Autodesk Inventor part; units mm, degrees
ref_plane "YZ Plane" through (0, 0, 0) normal (1, 0, 0) x (0, 1, 0)
ref_plane "XZ Plane" through (0, 0, 0) normal (0, 1, 0) x (-1, 0, 0)
ref_plane "XY Plane" through (0, 0, 0) normal (0, 0, 1) x (1, 0, 0)
sketch "Sketch1" plane through (0, 0, 0) normal (0, 0, 1) x (1, 0, 0)
  circle A0 centre (0, 0) radius 37.7825
  dimension "d0" = 75.565
extrude "Extrusion1" add sketch "Sketch1" against normal blind 6.35
sketch "Sketch2" plane through (0, 0, 0) normal (0, 0, 1) x (1, 0, 0)
  line L0 (-31.115, -10.4775) -> (31.115, -10.4775)
  line L1 (31.115, -10.4775) -> (31.115, -17.6657)
  line L2 (31.115, -17.6657) -> (-31.115, -17.6657)
  line L3 (-31.115, -17.6657) -> (-31.115, -10.4775)
  line L4 (-31.115, 15.5575) -> (31.115, 15.5575)
  line L5 (31.115, 15.5575) -> (31.115, 10.4775)
  line L6 (31.115, 10.4775) -> (-31.115, 10.4775)
  line L7 (-31.115, 10.4775) -> (-31.115, 15.5575)
  point P0 (0, 0)
  point P1 (31.115, -14.0716)
  point P2 (31.115, 13.0175)
  dimension "d3" = 7.1882
  dimension "d4" = 62.23
  dimension "d5" = 31.115
  dimension "d6" = 10.4775
  dimension "d10" = 62.23
  dimension "d11" = 31.115
  dimension "d12" = 10.4775
  dimension "d13" = 5.08
extrude "Extrusion2" add sketch "Sketch2" along normal blind 119.38
fillet "Fillet1" radius 3.175 5 edges at (-31.115, -14.0716, 119.38) (31.115, -14.0716, 119.38) (31.115, -17.6657, 59.69) (-31.115, -17.6657, 59.69) (0, -17.6657, 119.38)
fillet "Fillet2" radius 3.175 5 edges at (-31.115, 13.0175, 119.38) (31.115, 13.0175, 119.38) (-31.115, 15.5575, 59.69) (0, 15.5575, 119.38) (31.115, 15.5575, 59.69)
sketch "Sketch3" plane through (-31.115, -10.4775, 0) normal (0, 1, 0) x (1, 0, 0)
  line L0 (0, -116.205) -> (0, 0)
  line L1 (59.055, -119.38) -> (3.175, -119.38)
  line L2 (62.23, 0) -> (62.23, -116.205)
  line L3 (59.055, 0) -> (3.175, 0)
  point P0 (31.115, 0)
  point P1 (7.5438, -111.8362)
  point P2 (7.5438, -7.5438)
  point P3 (54.6862, -7.5438)
  point P4 (54.6862, -111.8362)
  dimension "d15" = 7.5438
  dimension "d16" = 7.5438
  dimension "d17" = 7.5438
  dimension "d18" = 7.5438
  dimension "d19" = 7.5438
  dimension "d20" = 7.5438
  dimension "d21" = 7.5438
  dimension "d22" = 7.5438
hole "Hole1" at (-23.5712, -10.4775, 111.8362) at (-23.5712, -10.4775, 7.5438) at (23.5712, -10.4775, 7.5438) at (23.5712, -10.4775, 111.8362) direction (0, -1, 0) diameter 5.842 end through all
sketch "Sketch4" plane through (-31.115, 10.4775, 0) normal (0, -1, 0) x (1, 0, 0)
  circle A0 centre (54.6862, 111.8362) radius 2.1717
  circle A1 centre (54.6862, 7.5362) radius 2.1717
  circle A2 centre (7.5362, 7.5362) radius 2.1717
  circle A3 centre (7.5362, 111.8362) radius 2.1717
  point P0 (31.115, 0)
hole "Hole2" at (23.5712, 10.4775, 111.8362) at (-23.5788, 10.4775, 111.8362) at (-23.5788, 10.4775, 7.5362) at (23.5712, 10.4775, 7.5362) direction (0, 1, 0) diameter 4.4958 end through all
sketch "Sketch5" plane through (0, 0, -6.35) normal (0, 0, -1) x (-1, 0, 0)
  circle A0 centre (0, 27.305) radius 2.921
  arc A1 (-0.6096, -25.2301) -> (-0.6096, -29.3799) centre (0, -27.305) ccw
  point P0 (0, 0)
hole "Hole3" at (0, 27.305, -6.35) at (0, -27.305, -6.35) direction (0, 0, 1) diameter 4.4958 end through all
sketch "Sketch7" plane through (0, 0, -6.35) normal (0, 0, -1) x (-1, 0, 0)
  line L0 (21.939, 20) -> (25.939, 20)
  line L1 (25.939, 20) -> (25.939, -20)
  line L2 (25.939, -20) -> (21.939, -20)
  line L3 (21.939, -20) -> (21.939, 20)
  line L4 (22.439, -16.8541) -> (22.439, 16.8541)
  line L5 (25.439, 16.8541) -> (25.439, -16.8541)
  point P0 (0, 0)
  point P1 (23.939, -20)
  point P2 (23.939, 20)
  dimension "d51" = 4
  dimension "d53" = 0.5
  dimension "d54" = 40
  dimension "d55" = 20
extrude "Extrusion4" cut sketch "Sketch7" against normal blind 3
sketch "Sketch8" plane through (0, 0, -6.35) normal (0, 0, -1) x (-1, 0, 0)
  line L0 (27.94, 15.5575) -> (-27.94, 15.5575)
  line L1 (-20.1422, 20.5105) -> (-13.7922, 20.5105)
  line L2 (-13.7922, 20.5105) -> (-13.7922, 17.3355)
  line L3 (-13.7922, 17.3355) -> (-20.1422, 17.3355)
  line L4 (-20.1422, 17.3355) -> (-20.1422, 20.5105)
  line L5 (-20.1422, 20.3225) -> (-20.1422, 16.7818)
  point P0 (0, 0)
  dimension "d58" = 6.35
  dimension "d59" = 3.175
  dimension "d60" = 0
  dimension "d61" = 1.778
extrude "Extrusion5" cut sketch "Sketch8" against normal through all
sketch "Sketch9" plane through (-27.94, 15.5575, 0) normal (0, 1, 0) x (1, 0, 0)
  line L0 (41.7322, -0.635) -> (48.0822, -0.635)
  line L1 (48.0822, -0.635) -> (48.0822, -3.81)
  line L2 (48.0822, -3.81) -> (41.7322, -3.81)
  line L3 (41.7322, -3.81) -> (41.7322, -0.635)
  line L4 (-9.8425, 0) -> (65.7225, 0)
  point P0 (27.94, 0)
  point P1 (41.7322, 0)
  point P2 (48.0822, 0)
  point P3 (48.0822, -2.2225)
  dimension "d64" = 0
  dimension "d66" = 0
  dimension "d67" = 0.635
  dimension "d68" = 3.175
extrude "Extrusion6" cut sketch "Sketch9" against normal up to next
sketch "Sketch10" plane through (0, 0, 0) normal (0, 0, 1) x (1, 0, 0)
  line L0 (33.2105, 1.5875) -> (36.3855, 1.5875)
  line L1 (36.3855, 1.5875) -> (36.3855, -1.5875)
  line L2 (36.3855, -1.5875) -> (33.2105, -1.5875)
  line L3 (33.2105, -1.5875) -> (33.2105, 1.5875)
  circle A0 centre (0, 0) radius 37.7825
  line L4 (36.2585, 1.4605) -> (33.3375, 1.4605)
  line L5 (33.3375, 1.4605) -> (33.3375, -1.4605)
  line L6 (33.3375, -1.4605) -> (36.2585, -1.4605)
  line L7 (36.2585, -1.4605) -> (36.2585, 1.4605)
  dimension "d71" = 3.175
  dimension "d72" = 3.175
  dimension "d73" = 36.3855
  dimension "d74" = 37.7825
  dimension "d75" = 0.127
  dimension "d79" = 1.5875
extrude "Extrusion7" add sketch "Sketch10" along normal blind 6.35 contours L7 L6 L5 L4
fillet "Fillet4" radius 1 4 edges at (33.3375, 1.4605, 3.175) (36.2585, 1.4605, 3.175) (36.2585, -1.4605, 3.175) (33.3375, -1.4605, 3.175)
equation "\"d10\" = d4"
properties part number "Supportv2_3dprinted" material "ABS Plastic"
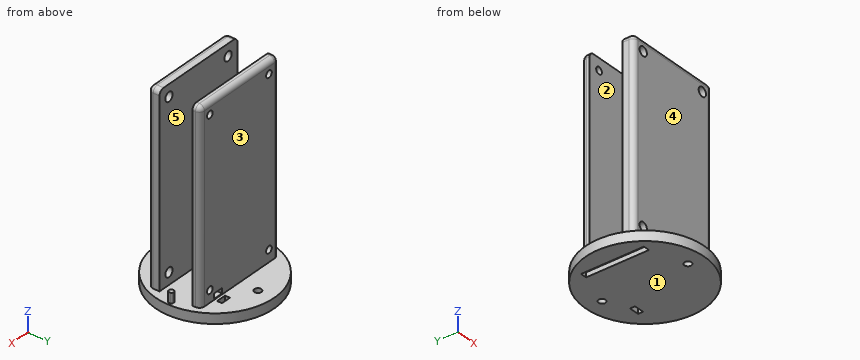
The listing builds one solid part. Answer for the finished solid, in the listing's coordinates (mm). Face numbers are marked on the shaded views. A direction names the side the tool comes from. Round coordinates to 2 decimals unless told otherwise and drop trailing zeros. Write each loop counter-clockwise with the first axis right and the second up, starting at its lowest first coordinate (ties: lowest second). Pieces come first, ordered by that corner, then holes. Notation, with made-up numbers: M 18,11.25 L 75,11.25 A12 ccw 75,26.25 Z; hole C 63.5,-24 d11. An arc over 180 degrees is marked long. Write each question's results on one line, items separated by ' | '. Start each with the question number.
Item 1: A cutting plane is placed at B-B on x = 0. State how many separate pieces and enclosed holes the cut face has, and give its area (3 significant figures).
Item 2: Flat-ended cylindrical pins translate along their axes: pin 1 Ø8 at (x, z) = (14.5, 21) entering from +Y; pin 2 Ø2 at (y, z) = (11.5, 40.5) entering from +X (3 decimals); pin 3 Ø3.5 at (y, z) = (-10, -4.5) entering from -X. Find the tip coordinate at first contact, or state that the pin passes through.
Item 3: A cutting plane is placed at D-D on y = -12.5. Write down the section's boundary in (x, z) (3 decimals), and give its area (3 significant figures).
Item 4: For the marked faces 4 and 5, determine the directions among +Z, -Z, +X, -X, +Y, -Y from which every point of the face is accessible in a straight line to the end or side of a thin tool.
Item 5: Straight lines are drawn through the part: L1, parallel to Y at x = 0, z = -2.75; L2, parallel to Y at x = -2, z = 74; L3, parallel to Z at x = 19.5, y = -26.5. For each, find the intervals that lie inside material, in ascending order. Write a range as [from, to].
Item 6: For a pull along Y with two mould halves and no side action, classify the marked faces 1, 2 and 3 as pulls with the +Y half, pulls with the -Y half, needs draft (parallel to the pull), parting line crosses it, or undercut.
Item 7: A cutting plane is placed at C-C on y = 27.5. Write down the section's boundary in (x, z).
Check sheet entries:
1) separate pieces: 3 | enclosed holes: 0 | area: 1,880 mm²
2) pin 1: y = 15.56 | pin 2: x = 31.115 | pin 3: x = -36.87
3) outline: M -35.655,-6.35 L -25.939,-6.35 L -25.939,-3.35 L -21.939,-3.35 L -21.939,-6.35 L 35.655,-6.35 L 35.655,0 L 31.115,0 L 31.115,116.205 A3.175 ccw 27.94,119.38 L -27.94,119.38 A3.175 ccw -31.115,116.205 L -31.115,0 L -35.655,0 Z; hole C -23.571,7.544 d5.842; hole C -23.571,111.836 d5.842; hole C 23.571,7.544 d5.842; hole C 23.571,111.836 d5.842 | area: 7,760 mm²
4) face 4: +Z, +X, -X, -Y | face 5: +Z, +X, -X
5) L1: [-37.78, -29.55], [-25.06, 25.06], [29.55, 37.78] | L2: [-17.67, -10.48], [10.48, 15.56] | L3: [-6.35, 0]
6) face 1: needs draft | face 2: undercut | face 3: pulls with the +Y half
7) outline: M -25.91,-6.35 L -2.24,-6.35 L -2.24,0 L -25.91,0 Z; M 2.24,-6.35 L 25.91,-6.35 L 25.91,0 L 2.24,0 Z
